Geometry: see drawing. Coordinates: mm, zero at the bounding-box minimum. A direction names the side the tool comes from. Round coordinates to 2 decimals unless told otherwise and drop trailing zeros. Write each loop counter-clockwise with the first axis right and the second up, starting at its lowest first coordinate (ties: lowest second). Pieces come first, ordered by that corner, then holes.
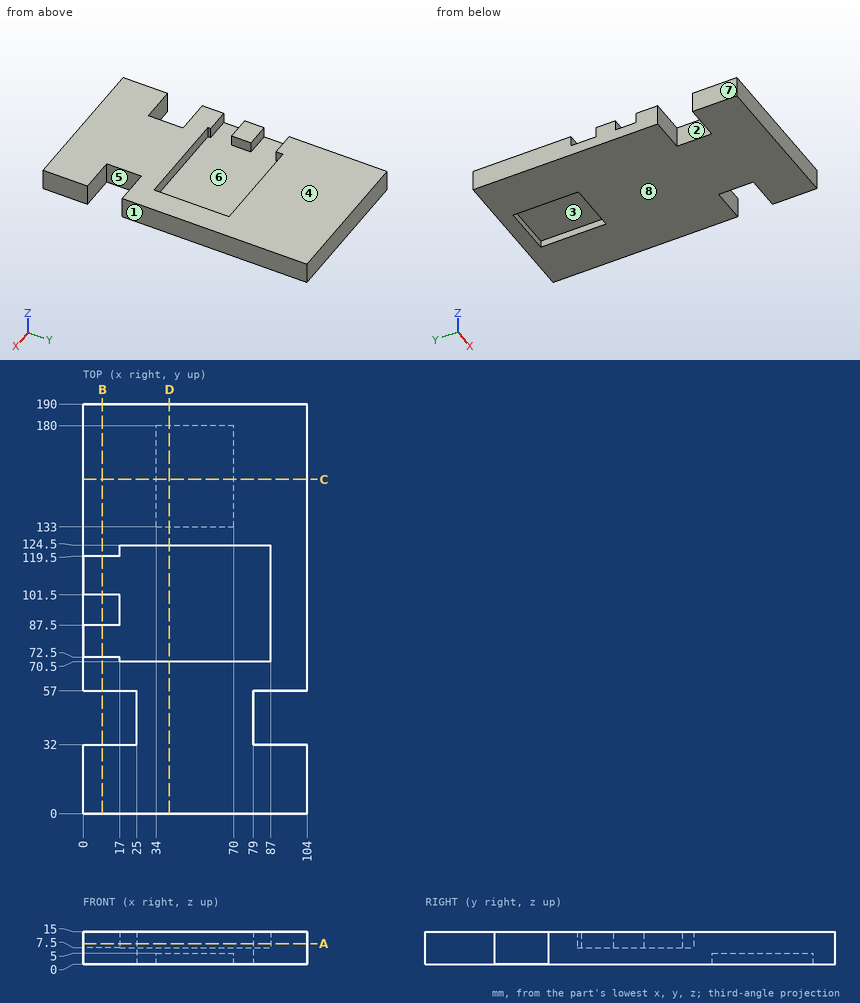
1) Section query A-A on z = 9.5. Return the cut outline in (x, y).
Taken from the geometry:
outline: (0, 0) - (104, 0) - (104, 32) - (79, 32) - (79, 57) - (104, 57) - (104, 190) - (0, 190) - (0, 119.5) - (17, 119.5) - (17, 124.5) - (87, 124.5) - (87, 70.5) - (17, 70.5) - (17, 72.5) - (0, 72.5) - (0, 57) - (25, 57) - (25, 32) - (0, 32) - close; (0, 87.5) - (17, 87.5) - (17, 101.5) - (0, 101.5) - close
2) Reachability of the marked faces 1, 2, 3, 4 and 5 from +Z, -Z, +X, -X, +Y, -Y: full face, straight path, thin tool, end or side. Return the list, or none.
Taken from the geometry:
face 1: +Z, -Z, +X, +Y, -Y
face 2: +Z, -Z, -X
face 3: -Z
face 4: +Z, +X, -X, +Y, -Y
face 5: +Z, -Z, +X
3) Section query C-C on y = 155. Return the cut outline in (x, z), then the cut area to 3 significant figures.
Taken from the geometry:
outline: (0, 0) - (34, 0) - (34, 5) - (70, 5) - (70, 0) - (104, 0) - (104, 15) - (0, 15) - close
area: 1,380 mm2
4) Contact query for flat-ended pins moving along their axis: P1, Ø16, axis at x = 23, y = 109.5, coming from the +Z side; P2, Ø2, axis at y = 34, z = 5.5, coming from the +X side; P3, Ø7.5, axis at y = 44.5, z = 9, coming from the -X side. Output: stop coordinate, or through.
Taken from the geometry:
P1: stops at z = 7.5
P2: stops at x = 79
P3: stops at x = 25
5) Material intervals for line 1 (Y direction, x = 50, z = 12); line 2 (Y direction, x = 91.5, z = 7.75); line 3 (X direction, y = 147.5, z = 2), sorted ascending.
Taken from the geometry:
line 1: y = 0 to 70.5, 124.5 to 190
line 2: y = 0 to 32, 57 to 190
line 3: x = 0 to 34, 70 to 104
6) Section query B-B on x = 9. Return the cut outline in (y, z), then the cut area to 3 significant figures.
Taken from the geometry:
outline: (0, 0) - (32, 0) - (32, 15) - (0, 15) - close; (57, 0) - (190, 0) - (190, 15) - (119.5, 15) - (119.5, 7.5) - (101.5, 7.5) - (101.5, 15) - (87.5, 15) - (87.5, 7.5) - (72.5, 7.5) - (72.5, 15) - (57, 15) - close
area: 2,230 mm2
7) Section query D-D on x = 40. Return the cut outline in (y, z), then the cut area to 3 significant figures.
Taken from the geometry:
outline: (0, 0) - (133, 0) - (133, 5) - (180, 5) - (180, 0) - (190, 0) - (190, 15) - (124.5, 15) - (124.5, 7.5) - (70.5, 7.5) - (70.5, 15) - (0, 15) - close
area: 2,210 mm2
8) Pull-direction query (X, two-part tool) for the marked faces 6, 7 and 8; classes: released by +X, released by -X, zero draft, split by the parting line, or undercut.
Taken from the geometry:
face 6: undercut
face 7: released by -X
face 8: zero draft
